Read the model definition and answer for the solid it produces. Units are mm, in the model's axes. Coordinates: 2 decimals unless noted, no trailing zeros. Loops run counter-clockwise (first coordinate to the right, second up) from the corner with the lowest first, then second, coordinate; pieces in that order, holes last. Notation, with made-up numbers: M -11,52 L 29,52 A23 cw 29,91 Z; hole C 7,8 d9. An arc over 180 degrees is marked long. Put each result on its own line as item: value.
from build123d import *

# Parameters (mm, degrees)
F1_DEPTH = 5
F2_DEPTH = 10


with BuildPart() as f1:
    # F0 (on Top) → F1 (new body)
    with BuildSketch(Plane.XY):
        with BuildLine():
            Line((25.5, 0), (2, 0))
            ThreePointArc((2, 0), (1.414214, -1.414214), (0, -2))
            Line((0, -2), (27.5, -2))
            ThreePointArc((27.5, -2), (26.085786, -1.414214), (25.5, 0))
        make_face()
        with BuildLine():
            ThreePointArc((0, 2), (1.414214, 1.414214), (2, 0))
            Line((2, 0), (25.5, 0))
            ThreePointArc((25.5, 0), (26.085786, 1.414214), (27.5, 2))
            Line((27.5, 2), (0, 2))
        make_face()
        with BuildLine():
            Line((0, 0), (0, 2))
            ThreePointArc((0, 2), (-2, 0), (0, -2))
            Line((0, -2), (0, 0))
        make_face()
        with BuildLine():
            Line((55, 2), (27.5, 2))
            ThreePointArc((27.5, 2), (28.914214, 1.414214), (29.5, 0))
            Line((29.5, 0), (53, 0))
            ThreePointArc((53, 0), (53.585786, 1.414214), (55, 2))
        make_face()
        with BuildLine():
            ThreePointArc((29.5, 0), (28.914214, -1.414214), (27.5, -2))
            Line((27.5, -2), (55, -2))
            ThreePointArc((55, -2), (53.585786, -1.414214), (53, 0))
            Line((53, 0), (29.5, 0))
        make_face()
        with BuildLine():
            Line((82.5, 2), (55, 2))
            ThreePointArc((55, 2), (56.414214, 1.414214), (57, 0))
            Line((57, 0), (80.5, 0))
            ThreePointArc((80.5, 0), (81.085786, 1.414214), (82.5, 2))
        make_face()
        with BuildLine():
            ThreePointArc((57, 0), (56.414214, -1.414214), (55, -2))
            Line((55, -2), (82.5, -2))
            ThreePointArc((82.5, -2), (81.085786, -1.414214), (80.5, 0))
            Line((80.5, 0), (57, 0))
        make_face()
        with BuildLine():
            ThreePointArc((84.5, 0), (83.914214, 1.414214), (82.5, 2))
            Line((82.5, 2), (82.5, 0))
            Line((82.5, 0), (82.5, -2))
            ThreePointArc((82.5, -2), (83.914214, -1.414214), (84.5, 0))
        make_face()
    extrude(amount=F1_DEPTH)

    # F0 (on Top) → F2 (join)
    with BuildSketch(Plane.XY):
        with BuildLine():
            ThreePointArc((84.5, 0), (83.914214, 1.414214), (82.5, 2))
            Line((82.5, 2), (82.5, 0))
            Line((82.5, 0), (82.5, -2))
            ThreePointArc((82.5, -2), (83.914214, -1.414214), (84.5, 0))
        make_face()
        with BuildLine():
            Line((82.5, 0), (82.5, 2))
            ThreePointArc((82.5, 2), (81.085786, 1.414214), (80.5, 0))
            Line((80.5, 0), (82.5, 0))
        make_face()
        with BuildLine():
            ThreePointArc((80.5, 0), (81.085786, -1.414214), (82.5, -2))
            Line((82.5, -2), (82.5, 0))
            Line((82.5, 0), (80.5, 0))
        make_face()
        with BuildLine():
            ThreePointArc((53, 0), (53.585786, -1.414214), (55, -2))
            ThreePointArc((55, -2), (56.414214, -1.414214), (57, 0))
            Line((57, 0), (55, 0))
            Line((55, 0), (53, 0))
        make_face()
        with BuildLine():
            ThreePointArc((57, 0), (56.414214, 1.414214), (55, 2))
            ThreePointArc((55, 2), (53.585786, 1.414214), (53, 0))
            Line((53, 0), (55, 0))
            Line((55, 0), (57, 0))
        make_face()
        with BuildLine():
            Line((27.5, 0), (25.5, 0))
            ThreePointArc((25.5, 0), (26.085786, -1.414214), (27.5, -2))
            ThreePointArc((27.5, -2), (28.914214, -1.414214), (29.5, 0))
            Line((29.5, 0), (27.5, 0))
        make_face()
        with BuildLine():
            ThreePointArc((27.5, 2), (26.085786, 1.414214), (25.5, 0))
            Line((25.5, 0), (27.5, 0))
            Line((27.5, 0), (29.5, 0))
            ThreePointArc((29.5, 0), (28.914214, 1.414214), (27.5, 2))
        make_face()
        with BuildLine():
            ThreePointArc((0, -2), (1.414214, -1.414214), (2, 0))
            Line((2, 0), (0, 0))
            Line((0, 0), (0, -2))
        make_face()
        with BuildLine():
            Line((0, 0), (0, 2))
            ThreePointArc((0, 2), (-2, 0), (0, -2))
            Line((0, -2), (0, 0))
        make_face()
        with BuildLine():
            Line((0, 0), (2, 0))
            ThreePointArc((2, 0), (1.414214, 1.414214), (0, 2))
            Line((0, 2), (0, 0))
        make_face()
    extrude(amount=F2_DEPTH)


solid = f1.part
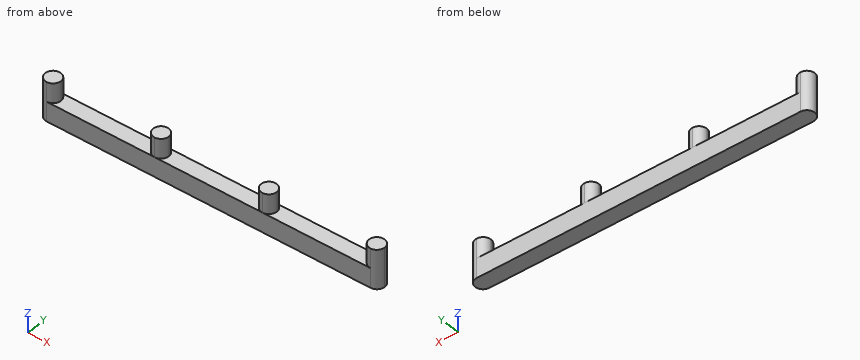
1) Find section A-A, the plane z = 9.25. Write down the section's boundary in (x, y), plus the area to 3 significant figures.
Answer list:
outline: M 0,-2 A2 ccw 2,0 A2 ccw 0,2 A2 ccw Z; M 25.5,0 A2 ccw 27.5,-2 A2 ccw 29.5,0 A2 ccw 27.5,2 A2 ccw Z; M 53,0 A2 ccw 55,-2 A2 ccw 57,0 A2 ccw 55,2 A2 ccw Z; M 80.5,0 A2 ccw 82.5,-2 A2 ccw 84.5,0 A2 ccw 82.5,2 A2 ccw Z
area: 50.3 mm^2
2) Find section C-C, the plane x = 22. Write down the section's boundary in (y, z), plus the area to 3 significant figures.
Answer list:
outline: M -2,0 L 2,0 L 2,5 L -2,5 Z
area: 20.0 mm^2
3) Straight lines are drawn through the part: line 1 (X direction, y = -0.2, z = 6.25); line 2 (X direction, y = -0.85, z = 7); line 3 (Z direction, x = 4, y = -1.3). For each, find the intervals that lie inside material, in ascending order. Write a range as [from, to].
Answer list:
line 1: x = [-1.99, 1.99], [25.51, 29.49], [53.01, 56.99], [80.51, 84.49]
line 2: x = [-1.81, 1.81], [25.69, 29.31], [53.19, 56.81], [80.69, 84.31]
line 3: z = [0, 5]
4) Given pin 1 Ø1.2 at (x, y) = (72, 0.5) entering from +Z; pin 2 Ø1 at (x, y) = (58.5, 0) entering from -Z, each flat-ended and moving along its own axis, determine where each tip first touches the part or whether it passes through.
Answer list:
pin 1: stops at z = 5
pin 2: stops at z = 0
5) Find section B-B, the plane y = 1.3. Write down the section's boundary in (x, z).
Answer list:
outline: M -1.52,0 L 84.02,0 L 84.02,10 L 80.98,10 L 80.98,5 L 56.52,5 L 56.52,10 L 53.48,10 L 53.48,5 L 29.02,5 L 29.02,10 L 25.98,10 L 25.98,5 L 1.52,5 L 1.52,10 L -1.52,10 Z
